from build123d import *

# Parameters (mm, degrees)
SKETCH1_R           = 37.5
SKETCH1_R_2         = 15
BOSS_EXTRUDE1_DEPTH = 5
SKETCH2_R           = 37.5
SKETCH2_R_2         = 30
BOSS_EXTRUDE2_DEPTH = 5
SKETCH3_R           = 1.65
CUT_EXTRUDE1_DEPTH  = 54.268189382
SKETCH4_R           = 3.1
CUT_EXTRUDE2_DEPTH  = 2
BOSS_EXTRUDE3_DEPTH = 10
SKETCH6_W           = 10
SKETCH6_H           = 60
BOSS_EXTRUDE4_DEPTH = 70
SKETCH7_R           = 13.5
CUT_EXTRUDE3_DEPTH  = 70
BOSS_EXTRUDE6_DEPTH = 10
SKETCH12_W          = 10
SKETCH12_H          = 8.531115437
BOSS_EXTRUDE7_DEPTH = 10
FILLET2_R           = 5
SKETCH10_R          = 1.65
CUT_EXTRUDE5_DEPTH  = 15
CHAMFER1_SIZE       = 10
FILLET3_R           = 2


# Read off the part's stored shape, not the designer's step: Boss-Extrude3
with BuildPart() as part:
    # Sketch1 → Boss-Extrude1 (new body)
    with BuildSketch(Plane(origin=(0, 0, 0), x_dir=(1, 0, 0), z_dir=(0, 1, 0))):
        with Locations(Location((0, 0, 0), (0, 0, 270))):
            Circle(SKETCH1_R)
        with Locations(Location((0, 0, 0), (0, 0, 270))):
            Circle(SKETCH1_R_2, mode=Mode.SUBTRACT)
    extrude(amount=BOSS_EXTRUDE1_DEPTH)

    # Sketch2 → Boss-Extrude2 (add)
    with BuildSketch(Plane(origin=(0, 5, 0), x_dir=(1, 0, 0), z_dir=(0, 1, 0))):
        with Locations(Location((0, 0, 0), (0, 0, 270))):
            Circle(SKETCH2_R)
        with Locations(Location((0, 0, 0), (0, 0, 270))):
            Circle(SKETCH2_R_2, mode=Mode.SUBTRACT)
    extrude(amount=BOSS_EXTRUDE2_DEPTH)

    # Sketch3 → Cut-Extrude1 (cut, through all)
    with BuildSketch(Plane(origin=(0, 5, 0), x_dir=(1, 0, 0), z_dir=(0, 1, 0))):
        with Locations(Location((0, -20, 0), (0, 0, 270))):
            Circle(SKETCH3_R)
        with Locations(Location((16.383040886, -11.471528727, 0), (0, 0, 270))):
            Circle(SKETCH3_R)
        with Locations(Location((-16.383040886, -11.471528727, 0), (0, 0, 270))):
            Circle(SKETCH3_R)
        with Locations(Location((-16.383040886, 11.471528727, 0), (0, 0, 90))):
            Circle(SKETCH3_R)
        with Locations(Location((0, 20, 0), (0, 0, 90))):
            Circle(SKETCH3_R)
        with Locations(Location((16.383040886, 11.471528727, 0), (0, 0, 90))):
            Circle(SKETCH3_R)
    extrude(amount=-CUT_EXTRUDE1_DEPTH, mode=Mode.SUBTRACT)

    # Sketch4 → Cut-Extrude2 (cut)
    with BuildSketch(Plane(origin=(0, 5, 0), x_dir=(1, 0, 0), z_dir=(0, 1, 0))):
        with Locations(Location((0, -20, 0), (0, 0, 270))):
            Circle(SKETCH4_R)
        with Locations(Location((16.383040886, -11.471528727, 0), (0, 0, 270))):
            Circle(SKETCH4_R)
        with Locations(Location((-16.383040886, -11.471528727, 0), (0, 0, 270))):
            Circle(SKETCH4_R)
        with Locations(Location((-16.383040886, 11.471528727, 0), (0, 0, 90))):
            Circle(SKETCH4_R)
        with Locations(Location((16.383040886, 11.471528727, 0), (0, 0, 90))):
            Circle(SKETCH4_R)
        with Locations(Location((0, 20, 0), (0, 0, 90))):
            Circle(SKETCH4_R)
    extrude(amount=-CUT_EXTRUDE2_DEPTH, mode=Mode.SUBTRACT)

    # Boss-Extrude3 outline → Boss-Extrude3 (add)
    with BuildSketch(Plane(origin=(0, 0, 0), x_dir=(1, 0, 0), z_dir=(0, 1, 0))):
        with BuildLine():
            Line((22.5, -30), (47.5, -30))
            Line((47.5, -30), (47.5, 30))
            Line((47.5, 30), (22.5, 30))
            ThreePointArc((22.5, 30), (37.5, 0), (22.5, -30))
        make_face()
    extrude(amount=BOSS_EXTRUDE3_DEPTH)

    # Sketch6 → Boss-Extrude4 (add)
    with BuildSketch(Plane(origin=(0, 10, 0), x_dir=(1, 0, 0), z_dir=(0, 1, 0))):
        with Locations((42.5, 0)):
            Rectangle(SKETCH6_W, SKETCH6_H)
    extrude(amount=BOSS_EXTRUDE4_DEPTH)

    # Sketch7 → Cut-Extrude3 (cut)
    with BuildSketch(Plane.ZY.offset(-37.5)):
        with Locations((0, 65)):
            Circle(SKETCH7_R)
    extrude(amount=-CUT_EXTRUDE3_DEPTH, mode=Mode.SUBTRACT)

    # Sketch9 → Boss-Extrude6 (add)
    with BuildSketch(Plane(origin=(47.5, 0, 0), x_dir=(0, 0, -1), z_dir=(1, 0, 0))):
        with BuildLine():
            ThreePointArc((-30, 80), (0, 110), (30, 80))
            Line((30, 80), (-30, 80))
        make_face()
    extrude(amount=-BOSS_EXTRUDE6_DEPTH)

    # Sketch12 → Boss-Extrude7 (add)
    with BuildSketch(Plane(origin=(47.5, 0, 0), x_dir=(0, 0, -1), z_dir=(1, 0, 0))):
        with Locations((-35, 44.792740579)):
            Rectangle(SKETCH12_W, SKETCH12_H)
        with Locations((35, 44.792740579)):
            Rectangle(SKETCH12_W, SKETCH12_H)
    extrude(amount=-BOSS_EXTRUDE7_DEPTH)

    # Fillet2
    fillet2_edges = [part.edges().sort_by_distance(p)[0] for p in [
        (42.5, 49.058298297, 30),
        (42.5, 40.52718286, 30),
        (42.5, 40.52718286, -30),
        (42.5, 49.058298297, -30),
    ]]
    fillet(fillet2_edges, radius=FILLET2_R)

    # Sketch10 → Cut-Extrude5 (cut)
    with BuildSketch(Plane.ZY.offset(-37.5)):
        with Locations((0, 106)):
            Circle(SKETCH10_R)
        with Locations((35.507041555, 44.5)):
            Circle(SKETCH10_R)
        with Locations((-35.507041555, 44.5)):
            Circle(SKETCH10_R)
    extrude(amount=-CUT_EXTRUDE5_DEPTH, mode=Mode.SUBTRACT)

    # Chamfer1
    # the kernel refuses this chamfer: 10 mm, written as the material it adds along each edge
    with BuildSketch(Plane(origin=(37.5, 10, 30), x_dir=(0.027495876610586317, 0.9996219169112968, 0), z_dir=(0, 0, -1))) as chamfer1_piece_1_section:
        Polygon((CHAMFER1_SIZE * 0.999621916911, -CHAMFER1_SIZE * 0.0274958766106), (-CHAMFER1_SIZE * 0.0274958766106, -CHAMFER1_SIZE * 0.999621916911), (0, 0), align=None)
    chamfer1_piece_1 = extrude(amount=60, mode=Mode.PRIVATE)
    chamfer1_piece_1 = chamfer1_piece_1 - Plane(origin=(0, 13.349530392, 0), x_dir=(0, 0, 1), z_dir=(0, -1, 0)) * Cylinder(30, 160, mode=Mode.PRIVATE)
    add(chamfer1_piece_1)

    # Fillet3
    fillet3_edges = [part.edges().sort_by_distance(p)[0] for p in [
        (42.5, 40.52718286, 40),
        (42.5, 49.058298297, 40),
        (42.5, 49.058298297, -40),
        (42.5, 40.52718286, -40),
    ]]
    fillet(fillet3_edges, radius=FILLET3_R)


solid = part.part
Geometry: final body of the model. Coordinates: model frame, mm. A direction names the side the tool comes from. Coordinates: 2 decimals unless noted, no trailing zeros. Order: outer loops, then holes, each group sorted by start corner. A loop starts at its lowest first (then second) coordinate and runs counter-clockwise, first axis right, second up.
1) Ray query, probe 1 along Y at (x, z) = (44, 0); probe 2 along X at (y, z) = (7.6, 0); probe 3 along X at (y, z) = (103.5, -18). Return the intervals inside material, ascending.
Result sheet:
probe 1: y = 0 to 51.5, 78.5 to 104.35, 107.65 to 110
probe 2: x = -37.5 to -30, 30 to 47.5
probe 3: x = 37.5 to 47.5
2) Draft query along Y for faces 6 (the cylindrical face through (42.4, 104.4, -0.4)), 7 (the cylindrical face through (-17.31, 4.01, -14.43)), 8 (the flat face through (18, 3, -13)). Return one class per face: released by +Y, released by -Y, zero draft, split by the parting line, or undercut.
Result sheet:
face 6: undercut
face 7: zero draft
face 8: released by +Y
3) First-contact query: P1, Ø1.9, axis at x = -0.5, z = 21, coming from the +Y side; P2, Ø3, axis at x = 16.38, z = -11.47, coming from the +Y side; P3, Ø1, axis at y = 94.5, z = -7, coming from the -X side; P4, Ø3.5, axis at x = 40.5, z = 36, coming from the +Y side. Flat tips, straight axial feed; report the tip coordinate or a pass-through.
Result sheet:
P1: stops at y = 3
P2: passes through
P3: stops at x = 37.5
P4: stops at y = 49.11
4) Section D-D (z = -20). Return loops of the section in (x, y), then the cut area to 3 significant figures.
Result sheet:
outline: (-31.72, 0) - (-1.65, 0) - (-1.65, 3) - (-3.1, 3) - (-3.1, 5) - (-22.36, 5) - (-22.36, 10) - (-31.72, 10) - close; (1.65, 0) - (47.5, 0) - (47.5, 102.36) - (37.5, 102.36) - (37.5, 20) - (27.5, 10) - (22.36, 10) - (22.36, 5) - (3.1, 5) - (3.1, 3) - (1.65, 3) - close
area: 1,520 mm2
5) Section C-C (x = 39.5). Return loops of the section in (y, z).
Result sheet:
outline: (0, -30) - (35.53, -30) arc R5 cw to (40.53, -35) - (40.53, -38) arc R2 ccw to (42.53, -40) - (47.06, -40) arc R2 ccw to (49.06, -38) - (49.06, -35) arc R5 cw to (54.06, -30) - (80, -30) arc R30 ccw to (80, 30) - (54.06, 30) arc R5 cw to (49.06, 35) - (49.06, 38) arc R2 ccw to (47.06, 40) - (42.53, 40) arc R2 ccw to (40.53, 38) - (40.53, 35) arc R5 cw to (35.53, 30) - (0, 30) - close; hole circle Ø3.3 at (44.5, -35.51); hole circle Ø3.3 at (44.5, 35.51); hole circle Ø27 at (65, 0); hole circle Ø3.3 at (106, 0)
6) Section A-A (y = 65). Return loops of the section in (x, z), then the cut area to 3 significant figures.
Result sheet:
outline: (37.5, -30) - (47.5, -30) - (47.5, -13.5) - (37.5, -13.5) - close; (37.5, 13.5) - (47.5, 13.5) - (47.5, 30) - (37.5, 30) - close
area: 330 mm2
7) Set-up query: faces 1 (the flat face through (43, 40.527, -36)), 2 (the flat face through (43, 49.058, 37)), 3 (the cylindrical face through (14.772, 1.521, 11.114)), 4 (the flat face through (42, 67, -30)), 5 (the flat face through (-18, 3, 13)). Return all of +Z, -Z, +X, -X, +Y, -Y with unobstructed straight access to the full face (end or side cutting, diameter ignored); none if empty.
Result sheet:
face 1: -Z, +X, -X, -Y
face 2: +Z, +X, -X, +Y
face 3: +Y, -Y
face 4: -Z, +X, -X, +Y
face 5: +Y
8) Section B-B (x = 0). Return loops of the section in (y, z).
Result sheet:
outline: (0, -37.5) - (10, -37.5) - (10, -30) - (5, -30) - (5, -23.1) - (3, -23.1) - (3, -21.65) - (0, -21.65) - close; (0, -18.35) - (3, -18.35) - (3, -16.9) - (5, -16.9) - (5, -15) - (0, -15) - close; (0, 15) - (5, 15) - (5, 16.9) - (3, 16.9) - (3, 18.35) - (0, 18.35) - close; (0, 21.65) - (3, 21.65) - (3, 23.1) - (5, 23.1) - (5, 30) - (10, 30) - (10, 37.5) - (0, 37.5) - close
